Verification items for the finished model (mm, model axes). A direction names the side the tool comes from. Give positions to 0.01 mm unless a question says otherwise; leave off trailing zeros. Order: outer loops, then holes, each group sorted by start corner. A loop starts at its lowest first (then second) coordinate and runs counter-clockwise, first axis right, second up.
from build123d import *

# Parameters (mm, degrees)
SKETCH2_R           = 5.08
BOSS_EXTRUDE2_DEPTH = 41.91
SKETCH8_W           = 50.8
SKETCH8_H           = 177.8
BOSS_EXTRUDE3_DEPTH = 12.7
SKETCH14_R          = 1.5
SKETCH14_R_2        = 3.81
CUT_EXTRUDE5_DEPTH  = 30.94
SKETCH18_R          = 12.5
CUT_EXTRUDE6_DEPTH  = 3
SKETCH19_W          = 42.604525883
SKETCH19_H          = 46.988260705
CUT_EXTRUDE7_DEPTH  = 85.804
SKETCH20_R          = 3.81
CUT_EXTRUDE8_DEPTH  = 157.771189784
SKETCH21_R          = 12.5
CUT_EXTRUDE9_DEPTH  = 4
SKETCH23_W          = 50.8
SKETCH23_H          = 12.7
BOSS_EXTRUDE4_DEPTH = 127


with BuildPart() as part:
    # Sketch2 → Boss-Extrude2 (new body)
    with BuildSketch(Plane(origin=(0, 0, 0), x_dir=(-1, 0, 0), z_dir=(0, 1, 0))):
        with Locations(Location((0, 0, 0), (0, 0, 90))):
            Circle(SKETCH2_R)
    extrude(amount=BOSS_EXTRUDE2_DEPTH)

    # Sketch8 → Boss-Extrude3 (add)
    with BuildSketch(Plane(origin=(0, 41.91, 0), x_dir=(1, 0, 0), z_dir=(0, 1, 0))):
        with Locations((0, -65.27767655)):
            Rectangle(SKETCH8_W, SKETCH8_H)
    extrude(amount=BOSS_EXTRUDE3_DEPTH)

    # Sketch14 → Cut-Extrude5 (cut)
    with BuildSketch(Plane.XZ.offset(-41.91)):
        with Locations(Location((15.5, 144.27767655, 0), (0, 0, 270))):
            Circle(SKETCH14_R)
        with Locations(Location((0, 128.77767655, 0), (0, 0, 270))):
            Circle(SKETCH14_R_2)
        with Locations(Location((-15.5, 113.27767655, 0), (0, 0, 270))):
            Circle(SKETCH14_R)
        with Locations(Location((15.5, 113.27767655, 0), (0, 0, 270))):
            Circle(SKETCH14_R)
        with Locations(Location((-15.5, 144.27767655, 0), (0, 0, 270))):
            Circle(SKETCH14_R)
    extrude(amount=-CUT_EXTRUDE5_DEPTH, mode=Mode.SUBTRACT)

    # Sketch18 → Cut-Extrude6 (cut)
    with BuildSketch(Plane(origin=(0, 54.61, 0), x_dir=(1, 0, 0), z_dir=(0, 1, 0))):
        with Locations(Location((0, -128.77767655, 0), (0, 0, 270))):
            Circle(SKETCH18_R)
    extrude(amount=-CUT_EXTRUDE6_DEPTH, mode=Mode.SUBTRACT)

    # Sketch19 → Cut-Extrude7 (cut)
    with BuildSketch(Plane.ZY.offset(25.4)):
        with Locations((-1.112784187, 18.415869648)):
            Rectangle(SKETCH19_W, SKETCH19_H)
    extrude(amount=-CUT_EXTRUDE7_DEPTH, mode=Mode.SUBTRACT)

    # Sketch20 → Cut-Extrude8 (cut, through all)
    with BuildSketch(Plane.XZ.offset(-41.91)):
        with Locations(Location((0, 0, 0), (0, 0, 270))):
            Circle(SKETCH20_R)
    extrude(amount=-CUT_EXTRUDE8_DEPTH, mode=Mode.SUBTRACT)

    # Sketch21 → Cut-Extrude9 (cut)
    with BuildSketch(Plane(origin=(0, 54.61, 0), x_dir=(1, 0, 0), z_dir=(0, 1, 0))):
        with Locations(Location((0, 0, 0), (0, 0, 270))):
            Circle(SKETCH21_R)
    extrude(amount=-CUT_EXTRUDE9_DEPTH, mode=Mode.SUBTRACT)

    # Sketch23 → Boss-Extrude4 (add)
    with BuildSketch(Plane(origin=(0, 0, -23.62232345), x_dir=(-1, 0, 0), z_dir=(0, 0, -1))):
        with Locations((0, 48.26)):
            Rectangle(SKETCH23_W, SKETCH23_H)
    extrude(amount=BOSS_EXTRUDE4_DEPTH)


solid = part.part
(1) Go/stop test with flat-tipped pins: pin 1 (7 mm diameter, centred on x = 0, z = 0, fed in from +Y); pin 2 (22.5 mm diameter, centred on x = 0, z = 128.78, fed in from +Y); pin 3 (7.5 mm diameter, centred on x = -4, z = 4, fed in from +Y). Record where each tip stops, or that it passes through.
Solved:
pin 1: passes through
pin 2: stops at y = 51.61
pin 3: stops at y = 50.61
(2) Release check for a two-part mould opening along Z. For faces 1 (the cylindrical face through (0.55, 53.13, 116.29)), 2 (the flat face through (0, 41.91, 4)), 3 (the flat face through (0, 48, 154.178)), 4 (the flat face through (0, 48, -150.622)) record: pulls with the +Z half, pulls with the -Z half, needs draft (parallel to the pull), parting line crosses it, or undercut.
Solved:
face 1: undercut
face 2: needs draft
face 3: pulls with the +Z half
face 4: pulls with the -Z half
(3) Scan lines: line 1 (Z direction, x = -0.5, y = 43); line 2 (X direction, y = 52.7, z = 0); line 3 (Z direction, x = -2, y = 51.25). Record each from-to range of solid material in increasing order.
Solved:
line 1: z = -150.62 to -3.78, 3.78 to 125, 132.55 to 154.18
line 2: x = -25.4 to -12.5, 12.5 to 25.4
line 3: z = -150.62 to -12.34, 12.34 to 125.53, 132.02 to 154.18
(4) Section check A-A, the plane x = 0. Enter the section's corners in (y, z), then the cut area to 3 significant figures.
Solved:
outline: (41.91, -150.62) - (54.61, -150.62) - (54.61, -12.5) - (50.61, -12.5) - (50.61, -3.81) - (41.91, -3.81) - close; (41.91, 3.81) - (50.61, 3.81) - (50.61, 12.5) - (54.61, 12.5) - (54.61, 116.28) - (51.61, 116.28) - (51.61, 124.97) - (41.91, 124.97) - close; (41.91, 132.59) - (51.61, 132.59) - (51.61, 141.28) - (54.61, 141.28) - (54.61, 154.18) - (41.91, 154.18) - close
area: 3,560 mm2
(5) Set-up check for faces 5 (the flat face through (3, 50.61, 3)), 6 (the flat face through (25.4, 48, 4)): record each of +Z, -Z, +X, -X, +Y, -Y from which the full face is reachable in a straight line by a thin tool's end or side.
Solved:
face 5: +Y
face 6: +Z, -Z, +X, +Y, -Y
(6) Section check B-B, the plane z = 0. Enter the section's corners in (x, y).
Solved:
outline: (-25.4, 41.91) - (-3.81, 41.91) - (-3.81, 50.61) - (-12.5, 50.61) - (-12.5, 54.61) - (-25.4, 54.61) - close; (3.81, 41.91) - (25.4, 41.91) - (25.4, 54.61) - (12.5, 54.61) - (12.5, 50.61) - (3.81, 50.61) - close
